from build123d import *


with BuildPart() as part:
    # Sweep-Thin1: sweep along a path in Sketch3
    with BuildLine(Plane(origin=(0, 0, 0), x_dir=(1, 0, 0), z_dir=(0, 1, 0))) as sweep_thin1_path:
        Line((0, 0), (200, 0))
    # Sketch2 → Sweep-Thin1 (sweep)
    with BuildSketch(Plane(origin=(0, 0, 0), x_dir=(0, 0, -1), z_dir=(1, 0, 0))):
        with BuildLine():
            Line((4.5, 12.5), (-4.5, 12.5))
            ThreePointArc((-4.5, 12.5), (-10.156854249, 10.156854249), (-12.5, 4.5))
            Line((-12.5, 4.5), (-12.5, -4.5))
            ThreePointArc((-12.5, -4.5), (-10.156854249, -10.156854249), (-4.5, -12.5))
            Line((-4.5, -12.5), (4.5, -12.5))
            ThreePointArc((4.5, -12.5), (10.156854249, -10.156854249), (12.5, -4.5))
            Line((12.5, -4.5), (12.5, 4.5))
            ThreePointArc((12.5, 4.5), (10.156854249, 10.156854249), (4.5, 12.5))
        make_face()
        with BuildLine():
            Line((4.5, 9.5), (-4.5, 9.5))
            ThreePointArc((-4.5, 9.5), (-8.035533906, 8.035533906), (-9.5, 4.5))
            Line((-9.5, 4.5), (-9.5, -4.5))
            ThreePointArc((-9.5, -4.5), (-8.035533906, -8.035533906), (-4.5, -9.5))
            Line((-4.5, -9.5), (4.5, -9.5))
            ThreePointArc((4.5, -9.5), (8.035533906, -8.035533906), (9.5, -4.5))
            Line((9.5, -4.5), (9.5, 4.5))
            ThreePointArc((9.5, 4.5), (8.035533906, 8.035533906), (4.5, 9.5))
        make_face(mode=Mode.SUBTRACT)
    sweep(path=sweep_thin1_path.line)


solid = part.part
Work out the finished part from the listing and answer in its coordinate system (mm). A direction names the side the tool comes from. Give positions to 0.01 mm unless a question says otherwise; leave off trailing zeros. Order: outer loops, then holes, each group sorted by start corner. A loop starts at its lowest first (then second) coordinate and runs counter-clockwise, first axis right, second up. Notation, with made-up numbers: (33, -14.75) -> (59, -14.75) arc R12 ccw to (59, -10.75) -> close; hole circle Ø3 at (-17.75, -20.5). An arc over 180 degrees is marked (long way). One line per item, written item: value.
Item 1: A tool of negligible diameter and unlimited length cuts with its end or side. For faces 1 (the cylindrical face through (101.4, 8, -8.07)), 2 (the flat face through (101, -12.5, 0)), from which of +Z, -Z, +X, -X, +Y, -Y can it reach the whole face along a straight path? Write none if from no direction.
Answer sheet:
face 1: +X, -X
face 2: +Z, -Z, +X, -X, -Y
Item 2: Find section B-B, the plane z = 2. Give the vertices of the cut face in (x, y).
Answer sheet:
outline: (0, -12.5) -> (200, -12.5) -> (200, -9.5) -> (0, -9.5) -> close; (0, 9.5) -> (200, 9.5) -> (200, 12.5) -> (0, 12.5) -> close
Item 3: Straight lines are drawn through the part: probe 1 along Z at (x, y) = (142.5, 0.5); probe 2 along Y at (x, z) = (119.5, 6.25). For each, find the intervals that lie inside material, in ascending order.
Answer sheet:
probe 1: -12.5 to -9.5, 9.5 to 12.5
probe 2: -12.31 to -9.18, 9.18 to 12.31
Item 4: Determine the mould class of faces 3 (the cylindrical face through (101.4, -8.07, -8)), 4 (the flat face through (101, 0, 12.5)), 5 (the cylindrical face through (101.4, 10.094, -10.219)), 6 (the flat face through (101, 12.5, 0)) for opening direction Z: released by +Z, released by -Z, zero draft, split by the parting line, or undercut.
Answer sheet:
face 3: undercut
face 4: released by +Z
face 5: released by -Z
face 6: zero draft
Item 5: Find section A-A, the plane x = 186. Give the vertices of the cut face in (y, z).
Answer sheet:
outline: (-12.5, -4.5) arc R8 ccw to (-4.5, -12.5) -> (4.5, -12.5) arc R8 ccw to (12.5, -4.5) -> (12.5, 4.5) arc R8 ccw to (4.5, 12.5) -> (-4.5, 12.5) arc R8 ccw to (-12.5, 4.5) -> close; hole (-9.5, -4.5) arc R5 ccw to (-4.5, -9.5) -> (4.5, -9.5) arc R5 ccw to (9.5, -4.5) -> (9.5, 4.5) arc R5 ccw to (4.5, 9.5) -> (-4.5, 9.5) arc R5 ccw to (-9.5, 4.5) -> close
